CAD build for the part. Positions are in the model's coordinates, mm. Round coordinates to 2 decimals unless told otherwise and drop trailing zeros. Loops run counter-clockwise (first coordinate to the right, second up) from the corner with the lowest first, then second, coordinate; pieces in that order, holes last. Notation, with made-up numbers: (-37, -39.75) -> (-19, -39.75) arc R26 ccw to (-19, -9.75) -> close; hole circle Ø9 at (-36.5, -10.5). An arc over 180 degrees is marked (long way). Answer as CSV lines item,"result".
Autodesk Inventor part; units mm, degrees
ref_plane "YZ Plane" through (0, 0, 0) normal (1, 0, 0) x (0, 1, 0)
ref_plane "XZ Plane" through (0, 0, 0) normal (0, 1, 0) x (-1, 0, 0)
ref_plane "XY Plane" through (0, 0, 0) normal (0, 0, 1) x (1, 0, 0)
sketch "Sketch1" plane through (0, 0, 0) normal (0, 0, 1) x (1, 0, 0)
  circle A0 centre (0, 0) radius 214
  circle A1 centre (0, 0) radius 254
  dimension "d31" = 508
  dimension "d32" = 428
extrude "Plate1" add sketch "Sketch1" against normal blind 2
sketch "Sketch2" plane through (0, 0, 0) normal (0, 0, 1) x (1, 0, 0)
  circle A0 centre (0, 0) radius 214 construction
  circle A1 centre (0, 0) radius 254 construction
  line L0 (0, 254) -> (0, 214) construction
  circle A2 centre (0, 234) radius 6.5
  dimension "d33" = 13
extrude "Cut1" cut sketch "Sketch2" against normal blind 2
pattern_circular "Circular Pattern1" count 12 over 360 about axis through (0, 0, 0) along (0, 0, -1) of "Cut1"
equation "\"d31\" = Колесо_диам3_борт_ступицы"
equation "\"d32\" = Колесо_диам4_дно_ступицы"
equation "\"d34\" = Thickness"
equation "\"d15\" = Thickness"
equation "\"BendRadius\" = Thickness"
equation "\"BendReliefWidth\" = Thickness"
equation "\"BendReliefDepth\" = 0.5 * Thickness"
equation "\"CornerReliefSize\" = 4 * Thickness"
equation "\"MinimumRemnant\" = 2 * Thickness"
equation "\"TransitionRadius\" = BendRadius"
equation "\"JacobiRadiusSize\" = BendRadius"
equation "\"GapSize\" = Thickness"
properties part number "DMF2.0 01 45 Gear ring 5"
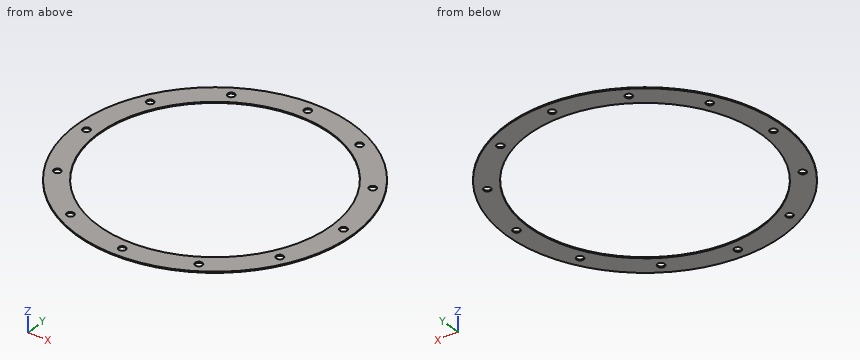
Q1. Drop flat-ended pins along their axis: pin 1 Ø1 at (x, z) = (178.5, -1) entering from +Y; pin 2 Ø21 at (x, y) = (-202.65, 117) entering from +Z. Give the stop position or say it passes through.
Results:
pin 1,"y = 181.2"
pin 2,"z = 0"
Q2. Slice it at A-A, the plane y = 59. Give the cut face in (x, z), and give its area (3 significant figures).
Results:
outline,"(-247.05, -2) -> (-205.71, -2) -> (-205.71, 0) -> (-247.05, 0) -> close; (205.71, -2) -> (247.05, -2) -> (247.05, 0) -> (205.71, 0) -> close"
area,"165 mm2"
Q3. Probe L1, parallel to X at y = -198, z = -0.15; L2, parallel to Y at x = -183, z = -1.05; L3, parallel to Y at x = 118.5, z = -1.05. List the from-to ranges inside material, lowest first. Write a range as [from, to].
Results:
L1,"[-159.1, -121.54], [-112.46, -81.19], [81.19, 112.46], [121.54, 159.1]"
L2,"[-176.14, -110.94], [110.94, 176.14]"
L3,"[-224.66, -208.97], [-196.33, -178.2], [178.2, 196.33], [208.97, 224.66]"
Q4. Slice it at C-C, the plane z = -0.9. Count the separate pieces of the cut face and the enclosed holes in it, and give its area (3 significant figures).
Results:
separate pieces,"1"
enclosed holes,"13"
area,"57,200 mm2"
Q5. Slice it at B-B, the plane x = 234. Give the cut face in (y, z), and give its area (3 significant figures).
Results:
outline,"(-98.79, -2) -> (-6.5, -2) -> (-6.5, 0) -> (-98.79, 0) -> close; (6.5, -2) -> (98.79, -2) -> (98.79, 0) -> (6.5, 0) -> close"
area,"369 mm2"
